For this review, take the finished solid that the model builds, in its own axes (mm). Coordinates: 2 decimals unless noted, no trailing zeros. Loops run counter-clockwise (first coordinate to the right, second up) from the corner with the lowest first, then second, coordinate; pieces in that order, holes last. Notation, with made-up numbers: (-38, 19) - (4, 19) arc R31 ccw to (4, 56) - close; hole circle Ø4 at (51.5, 72). An arc over 180 degrees is marked (long way). Use one line per item in the form item = value. Start each with the question number.
1. Draft analysis for pull direction X (two halves, no side actions). For faces 1 (the face through (-12.629, -19.925, 1.014)), 2 (the face through (46.074, -39.604, 0.986)), 3 (the face through (-51.17, -39.65, 0.99)), state which applies: +X half, -X half, draft (parallel to the pull), parting line (faces both ways), or undercut.
2. Add section A-A on x = -13. Give the boundary of the cut face in (y, z), and give its area (3 significant figures).
3. To check wall thickness, follow probe 1 along Y at (x, z) = (-28, 0.55); probe 2 along X at (y, z) = (14, 1.3); probe 3 along Y at (x, z) = (-44, 1.85). State the ranges of each line that lie inside material, in increasing order.
```python
from build123d import *

# Parameters (mm, degrees)
EXTRUDE_1_DEPTH     = 2
SKETCH_2_R          = 1.5
CUT_EXTRUDE_1_DEPTH = 2


with BuildPart() as part:
    # 草图1 → 凸台-拉伸1 (new body)
    with BuildSketch(Plane.XY):
        with BuildLine():
            Line((-49.07040619, 26.293617021), (43.92959381, 26.293617021))
            ThreePointArc((43.92959381, 26.293617021), (46.050914154, 25.414937365), (46.92959381, 23.293617021))
            Line((46.92959381, 23.293617021), (46.92959381, -37.506382979))
            ThreePointArc((46.92959381, -37.506382979), (46.050914154, -39.627703322), (43.92959381, -40.506382979))
            Line((43.92959381, -40.506382979), (-49.07040619, -40.506382979))
            ThreePointArc((-49.07040619, -40.506382979), (-51.191726533, -39.627703322), (-52.07040619, -37.506382979))
            Line((-52.07040619, -37.506382979), (-52.07040619, 23.293617021))
            ThreePointArc((-52.07040619, 23.293617021), (-51.191726533, 25.414937365), (-49.07040619, 26.293617021))
        make_face()
    extrude(amount=EXTRUDE_1_DEPTH)

    # 草图2 → 切除-拉伸1 (cut)
    with BuildSketch(Plane.XY.offset(2)):
        with Locations((-44.91440619, 14.101617021)):
            Circle(SKETCH_2_R)
        with Locations((43.22559381, 14.101617021)):
            Circle(SKETCH_2_R)
        with Locations((-44.91440619, -36.698382979)):
            Circle(SKETCH_2_R)
        with Locations((43.22559381, -36.698382979)):
            Circle(SKETCH_2_R)
        with Locations((-28.17040619, -3.745140574)):
            Circle(SKETCH_2_R)
        with Locations((-28.17040619, -18.594382979)):
            Circle(SKETCH_2_R)
        with Locations((-13.321163785, -3.745140574)):
            Circle(SKETCH_2_R)
        with Locations((-13.321163785, -18.594382979)):
            Circle(SKETCH_2_R)
    extrude(amount=-CUT_EXTRUDE_1_DEPTH, mode=Mode.SUBTRACT)


solid = part.part
```
Conclusion:
q1.face_1 = undercut
q1.face_2 = +X half
q1.face_3 = -X half
q2.outline = (-40.51, 0) - (-20.06, 0) - (-20.06, 2) - (-40.51, 2) - close; (-17.13, 0) - (-5.21, 0) - (-5.21, 2) - (-17.13, 2) - close; (-2.28, 0) - (26.29, 0) - (26.29, 2) - (-2.28, 2) - close
q2.area = 122 mm^2
q3.probe_1 = -40.51 to -20.08, -17.1 to -5.24, -2.25 to 26.29
q3.probe_2 = -52.07 to -46.41, -43.42 to 41.73, 44.72 to 46.93
q3.probe_3 = -40.51 to -37.89, -35.51 to 12.91, 15.29 to 26.29
